```python
from build123d import *

# Parameters (mm, degrees)
SKETCH1_W           = 142
SKETCH1_H           = 105
BOSS_EXTRUDE1_DEPTH = 2.5
CUT_EXTRUDE1_REACH  = 90.337
SKETCH2_R           = 1.6
SKETCH2_W           = 22
SKETCH2_H           = 93
FILLET1_R           = 13
FILLET2_R           = 2.5


with BuildPart() as part:
    # Sketch1 → Boss-Extrude1 (new body)
    with BuildSketch(Plane(origin=(0, 0, 0), x_dir=(1, 0, 0), z_dir=(0, 1, 0))):
        Rectangle(SKETCH1_W, SKETCH1_H)
    extrude(amount=BOSS_EXTRUDE1_DEPTH)

    # Sketch2 → Cut-Extrude1 (cut, up to next)
    with BuildSketch(Plane(origin=(0, 2.5, 0), x_dir=(1, 0, 0), z_dir=(0, 1, 0)), mode=Mode.PRIVATE) as cut_extrude1_sk1:
        with Locations(Location((-67.8, 49.3, 0), (0, 0, 270))):
            Circle(SKETCH2_R)
    cut_extrude1_tool1 = extrude(cut_extrude1_sk1.sketch, amount=-CUT_EXTRUDE1_REACH, mode=Mode.PRIVATE) & part.part
    # Sketch2 → Cut-Extrude1 (cut, up to next)
    with BuildSketch(Plane(origin=(0, 2.5, 0), x_dir=(1, 0, 0), z_dir=(0, 1, 0)), mode=Mode.PRIVATE) as cut_extrude1_sk2:
        with Locations(Location((0, 49.3, 0), (0, 0, 270))):
            Circle(SKETCH2_R)
    cut_extrude1_tool2 = extrude(cut_extrude1_sk2.sketch, amount=-CUT_EXTRUDE1_REACH, mode=Mode.PRIVATE) & part.part
    # Sketch2 → Cut-Extrude1 (cut, up to next)
    with BuildSketch(Plane(origin=(0, 2.5, 0), x_dir=(1, 0, 0), z_dir=(0, 1, 0)), mode=Mode.PRIVATE) as cut_extrude1_sk3:
        with Locations(Location((0, -49.3, 0), (0, 0, 270))):
            Circle(SKETCH2_R)
    cut_extrude1_tool3 = extrude(cut_extrude1_sk3.sketch, amount=-CUT_EXTRUDE1_REACH, mode=Mode.PRIVATE) & part.part
    # Sketch2 → Cut-Extrude1 (cut, up to next)
    with BuildSketch(Plane(origin=(0, 2.5, 0), x_dir=(1, 0, 0), z_dir=(0, 1, 0)), mode=Mode.PRIVATE) as cut_extrude1_sk4:
        with Locations(Location((-67.8, -49.3, 0), (0, 0, 270))):
            Circle(SKETCH2_R)
    cut_extrude1_tool4 = extrude(cut_extrude1_sk4.sketch, amount=-CUT_EXTRUDE1_REACH, mode=Mode.PRIVATE) & part.part
    # Sketch2 → Cut-Extrude1 (cut, up to next)
    with BuildSketch(Plane(origin=(0, 2.5, 0), x_dir=(1, 0, 0), z_dir=(0, 1, 0)), mode=Mode.PRIVATE) as cut_extrude1_sk5:
        with Locations(Location((67.8, 49.3, 0), (0, 0, 270))):
            Circle(SKETCH2_R)
    cut_extrude1_tool5 = extrude(cut_extrude1_sk5.sketch, amount=-CUT_EXTRUDE1_REACH, mode=Mode.PRIVATE) & part.part
    # Sketch2 → Cut-Extrude1 (cut, up to next)
    with BuildSketch(Plane(origin=(0, 2.5, 0), x_dir=(1, 0, 0), z_dir=(0, 1, 0)), mode=Mode.PRIVATE) as cut_extrude1_sk6:
        with Locations(Location((67.8, -49.3, 0), (0, 0, 270))):
            Circle(SKETCH2_R)
    cut_extrude1_tool6 = extrude(cut_extrude1_sk6.sketch, amount=-CUT_EXTRUDE1_REACH, mode=Mode.PRIVATE) & part.part
    # Sketch2 → Cut-Extrude1 (cut, up to next)
    with BuildSketch(Plane(origin=(0, 2.5, 0), x_dir=(1, 0, 0), z_dir=(0, 1, 0)), mode=Mode.PRIVATE) as cut_extrude1_sk7:
        with Locations((60, 0)):
            Rectangle(SKETCH2_W, SKETCH2_H)
    cut_extrude1_tool7 = extrude(cut_extrude1_sk7.sketch, amount=-CUT_EXTRUDE1_REACH, mode=Mode.PRIVATE) & part.part
    add(cut_extrude1_tool1.solids().sort_by_distance((-67.8, 2.5, -49.3))[0], mode=Mode.SUBTRACT)
    add(cut_extrude1_tool2.solids().sort_by_distance((0, 2.5, -49.3))[0], mode=Mode.SUBTRACT)
    add(cut_extrude1_tool3.solids().sort_by_distance((0, 2.5, 49.3))[0], mode=Mode.SUBTRACT)
    add(cut_extrude1_tool4.solids().sort_by_distance((-67.8, 2.5, 49.3))[0], mode=Mode.SUBTRACT)
    add(cut_extrude1_tool5.solids().sort_by_distance((67.8, 2.5, -49.3))[0], mode=Mode.SUBTRACT)
    add(cut_extrude1_tool6.solids().sort_by_distance((67.8, 2.5, 49.3))[0], mode=Mode.SUBTRACT)
    add(cut_extrude1_tool7.solids().sort_by_distance((60, 2.5, 0))[0], mode=Mode.SUBTRACT)

    # Fillet1
    fillet1_edges = [part.edges().sort_by_distance(p)[0] for p in [
        (49, 1.25, 46.5),
        (49, 1.25, -46.5),
    ]]
    fillet(fillet1_edges, radius=FILLET1_R)

    # Fillet2
    fillet2_edges = [part.edges().sort_by_distance(p)[0] for p in [
        (71, 1.25, 52.5),
        (71, 1.25, -52.5),
    ]]
    fillet(fillet2_edges, radius=FILLET2_R)


solid = part.part
```
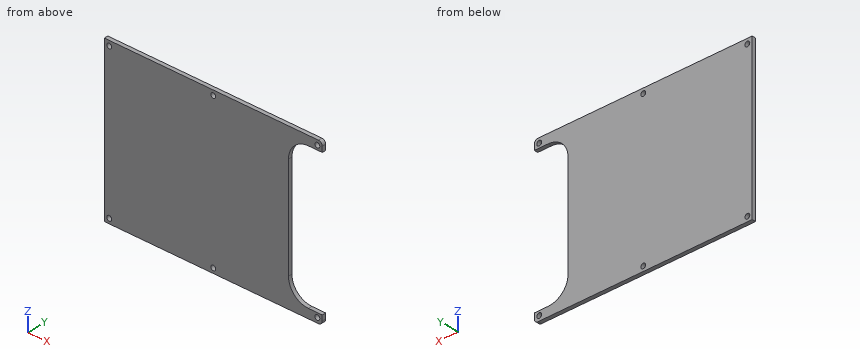
Read the model definition and answer for the solid it produces. Units are mm, in the model's axes. Coordinates: 2 decimals unless noted, no trailing zeros. Loops run counter-clockwise (first coordinate to the right, second up) from the corner with the lowest first, then second, coordinate; pieces in that order, holes last. Notation, with made-up numbers: (6.25, 87) - (10.25, 87) arc R22 ccw to (10.25, 100) - close; hole circle Ø11 at (25.25, -27.5). An arc over 180 degrees is marked (long way). Answer in a Markdown table with one row per item.
1. Find section B-B, the plane y = 0.5. Write down the section's boundary in (x, z), then the cut area to 3 significant figures.
Conclusion:
| item | result |
|---|---|
| outline | (-71, -52.5) - (68.5, -52.5) arc R2.5 ccw to (71, -50) - (71, -46.5) - (62, -46.5) arc R13 cw to (49, -33.5) - (49, 33.5) arc R13 cw to (62, 46.5) - (71, 46.5) - (71, 50) arc R2.5 ccw to (68.5, 52.5) - (-71, 52.5) - close; hole circle Ø3.2 at (-67.8, -49.3); hole circle Ø3.2 at (-67.8, 49.3); hole circle Ø3.2 at (0, -49.3); hole circle Ø3.2 at (0, 49.3); hole circle Ø3.2 at (67.8, -49.3); hole circle Ø3.2 at (67.8, 49.3) |
| area | 12,900 mm² |
2. Given pin 1 (0.8 mm diameter, centred on y = 1.5, z = 1.5, fed in from +X), flat-ended and moving along its own axis, determine where the tip first touches the part or whether it passes through.
Conclusion:
| item | result |
|---|---|
| pin 1 | stops at x = 49 |
3. Straight lines are drawn through the part: line 1 (X direction, y = 1.2, z = 49.3); line 2 (Z direction, x = -67.8, y = 0.6); line 3 (Z direction, x = 67.8, y = 0.75). For each, find the intervals that lie inside material, in ascending order.
Conclusion:
| item | result |
|---|---|
| line 1 | x = -71 to -69.4, -66.2 to -1.6, 1.6 to 66.2, 69.4 to 71 |
| line 2 | z = -52.5 to -50.9, -47.7 to 47.7, 50.9 to 52.5 |
| line 3 | z = -52.5 to -50.9, -47.7 to -46.5, 46.5 to 47.7, 50.9 to 52.5 |
4. Find section C-C, the plane z = 19.5. Write down the section's boundary in (x, y), then the cut area to 3 significant figures.
Conclusion:
| item | result |
|---|---|
| outline | (-71, 0) - (49, 0) - (49, 2.5) - (-71, 2.5) - close |
| area | 300 mm² |
5. Find section D-D, the plane z = -38. Write down the section's boundary in (x, y), then the cut area to 3 significant figures.
Conclusion:
| item | result |
|---|---|
| outline | (-71, 0) - (49.8, 0) - (49.8, 2.5) - (-71, 2.5) - close |
| area | 302 mm² |
6. Find section A-A, the plane x = -67.8. Write down the section's boundary in (y, z).
Conclusion:
| item | result |
|---|---|
| outline | (0, -52.5) - (2.5, -52.5) - (2.5, -50.9) - (0, -50.9) - close; (0, -47.7) - (2.5, -47.7) - (2.5, 47.7) - (0, 47.7) - close; (0, 50.9) - (2.5, 50.9) - (2.5, 52.5) - (0, 52.5) - close |
